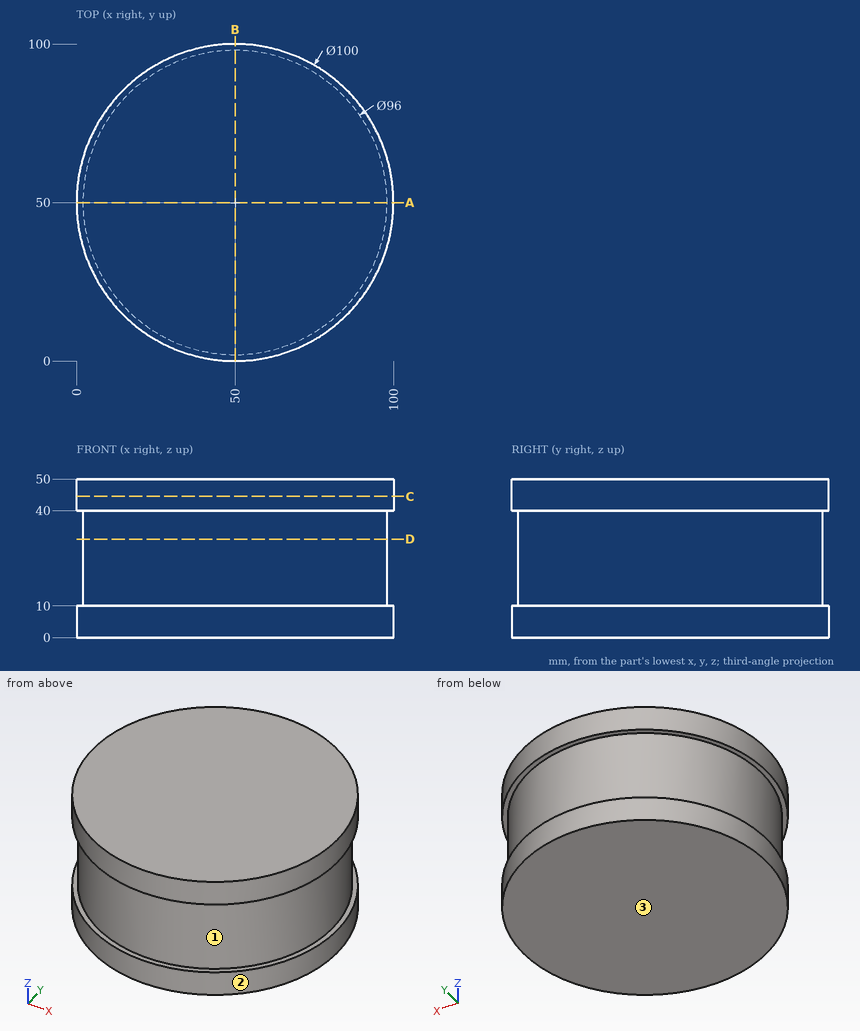
For this review, use the dimensioned drawing (mm, ordinates from the lowest corner) and the shaded views. Round coordinates to 2 decimals unless told otherwise and drop trailing zeros. Order: outer loops, then holes, each group sorted by start corner. A loop starts at its lowest first (then second) coordinate and runs counter-clockwise, first axis right, second up. Notation, with made-up numbers: (75.25, 67) - (103.25, 67) arc R29 ccw to (103.25, 97) - close; hole circle Ø7 at (32, -26). An arc over 180 degrees is marked (long way). Use one line per item in the form item = value.
Q1. Clearance check with flat-ended pins moving along their axes: P1, Ø6, axis at x = 29.5, z = 34.5, coming from the +Y side; P2, Ø6, axis at y = 48.5, z = 17, coming from the -X side; P3, Ø8, axis at x = 16, z = 30.5, coming from the +Y side. State where each tip first meets the part, or that it passes through.
Response values:
P1 = 94.7
P2 = 2
P3 = 87.47
Q2. Add section C-C on z = 44.5. Give the boundary of the cut face in (x, y), then the cut area to 3 significant figures.
Response values:
outline = circle Ø100 at (50, 50)
area = 7,850 mm^2
Q3. Add section D-D on z = 31. Give the boundary of the cut face in (x, y).
Response values:
outline = circle Ø96 at (50, 50)
Q4. Mouldability with a two-part tool opening along Z and no side actions: class the marked faces 1, 2 and 3 as pulls with the +Z half, pulls with the -Z half, needs draft (parallel to the pull), parting line crosses it, or undercut.
Response values:
face_1 = undercut
face_2 = needs draft
face_3 = pulls with the -Z half
Q5. Add section A-A on y = 50. Give the boundary of the cut face in (x, z).
Response values:
outline = (0, 0) - (100, 0) - (100, 10) - (98, 10) - (98, 40) - (100, 40) - (100, 50) - (0, 50) - (0, 40) - (2, 40) - (2, 10) - (0, 10) - close
Q6. To check wall thickness, follow line 1 (Y direction, x = 50, z = 23.5); line 2 (Y direction, x = 93, z = 8.5); line 3 (X direction, y = 58, z = 8.5). State the ranges of each line that lie inside material, in increasing order.
Response values:
line_1 = 2 to 98
line_2 = 24.49 to 75.51
line_3 = 0.64 to 99.36
